from build123d import *

# Parameters (mm, degrees)
SKETCH1_W           = 10
SKETCH1_H           = 2.9
REVOLVE1_ANGLE      = 359.999695921
BOSS_EXTRUDE1_START = -3
SKETCH2_W           = 10
SKETCH2_H           = 11
BOSS_EXTRUDE1_DEPTH = 7.5
BOSS_EXTRUDE2_START = 3.9
SKETCH3_W           = 40
SKETCH3_H           = 11
BOSS_EXTRUDE2_DEPTH = 4


with BuildPart() as part:
    # Sketch1 → Revolve1 (revolve)
    with BuildSketch(Plane.XY):
        with Locations((0, 4.55)):
            Rectangle(SKETCH1_W, SKETCH1_H)
    revolve(axis=Axis((-5, 0, 0), (1, 0, 0)), revolution_arc=REVOLVE1_ANGLE)

    # Sketch2 → Boss-Extrude1 (add)
    with BuildSketch(Plane(origin=(0, 0, 0), x_dir=(1, 0, 0), z_dir=(0, 1, 0)).offset(BOSS_EXTRUDE1_START)):
        with Locations((0, -9.5)):
            Rectangle(SKETCH2_W, SKETCH2_H)
    extrude(amount=BOSS_EXTRUDE1_DEPTH)

    # Sketch3 → Boss-Extrude2 (add)
    with BuildSketch(Plane(origin=(0, 0, 0), x_dir=(1, 0, 0), z_dir=(0, 1, 0)).offset(BOSS_EXTRUDE2_START)):
        with Locations((15, -14.5)):
            Rectangle(SKETCH3_W, SKETCH3_H)
    extrude(amount=BOSS_EXTRUDE2_DEPTH)


solid = part.part
Read the model definition and answer for the solid it produces. Units are mm, in the model's axes. Coordinates: 2 decimals unless noted, no trailing zeros. Loops run counter-clockwise (first coordinate to the right, second up) from the corner with the lowest first, then second, coordinate; pieces in that order, holes last.
Q1. The part is cut by section C-C on x = 31.5. Write down the section's boundary in (y, z).
Q2. The mould has two halves that part along Z. Classify faces 1 (the face through (0.1, -3.1, 0.1)), 2 (the face through (0, 0, 15)), 3 (the face through (0, -3, 10)), 4 (the face through (0, 4.5, 6)): +Z half, -Z half, draft (parallel to the pull), parting line (faces both ways), or undercut.
Q3. The part is cut by section D-D on y = 2.5. Write down the section's boundary in (x, z), and give its area (3 significant figures).
Q4. Each of these flat-tipped pins is pushed along its axis until it touches: pin 1 Ø3 at (y, z) = (-1.5, 12) entering from +X; pin 2 Ø1.5 at (x, z) = (22, 6.5) entering from +Y; pin 3 Ø4 at (x, z) = (0, 5.5) entering from +Y; pin 4 Ø8 at (x, z) = (1.5, 12.5) entering from -Y. Where does it stop, or does it pass through?
Q5. The part is cut by section B-B on z = 11.25. Write down the section's boundary in (x, y).
Q6. Consider probe 1 along Z at (x, y) = (2.25, 0); probe 2 along Y at (x, z) = (-1, 0.25); probe 3 along X at (y, z) = (2.5, 2.5). Determine where each line is inside the solid, lowest interval first.
Q7. The part is cut by section A-A on y = 0. Write down the section's boundary in (x, z).
Results below:
1. outline: (3.9, 9) - (7.9, 9) - (7.9, 20) - (3.9, 20) - close
2. face 1: undercut
2. face 2: +Z half
2. face 3: draft
2. face 4: undercut
3. outline: (-5, -5.45) - (5, -5.45) - (5, -1.83) - (-5, -1.83) - close; (-5, 1.83) - (5, 1.83) - (5, 15) - (-5, 15) - close
3. area: 168 mm2
4. pin 1: stops at x = 5
4. pin 2: passes through
4. pin 3: stops at y = 4.87
4. pin 4: stops at y = -3
5. outline: (-5, -3) - (5, -3) - (5, 3.9) - (35, 3.9) - (35, 7.9) - (-5, 7.9) - close
6. probe 1: z = -6 to -3.1, 3.1 to 15
6. probe 2: y = -5.99 to -3.09, 3.09 to 5.99
6. probe 3: x = -5 to 5
7. outline: (-5, -6) - (5, -6) - (5, -3.1) - (-5, -3.1) - close; (-5, 3.1) - (5, 3.1) - (5, 15) - (-5, 15) - close
